from build123d import *

# Parameters (mm, degrees)
SKETCH_1_W                 = 300
SKETCH_1_H                 = 30
EXTRUDE_1_DEPTH            = 20
SKETCH_3_R                 = 4
CUT_EXTRUDE_1_DEPTH        = 155.272486205
SKETCH_3_3_R               = 6
SKETCH_3_3_R_2             = 4
CUT_EXTRUDE_2_DEPTH        = 155.272486205
SKETCH_3_4_R               = 13.5
SKETCH_3_4_R_2             = 13.25
SKETCH_3_4_R_3             = 6
CUT_EXTRUDE_3_DEPTH        = 155.272486205
SKETCH_3_5_R               = 2.4
CUT_EXTRUDE_4_DEPTH        = 4.5
SKETCH_3_6_R               = 2.4
CUT_EXTRUDE_5_DEPTH        = 5
SKETCH_4_R                 = 5
EXTRUDE_2_DEPTH            = 28
SKETCH_5_R                 = 2.55
CUT_EXTRUDE_6_DEPTH        = 4
SKETCH_6_W                 = 8.216991224
SKETCH_6_H                 = 30
CUT_EXTRUDE_7_DEPTH        = 5
CHAMFER_1_SIZE             = 2
CHAMFER_1_OF_MIRROR_2_SIZE = 2


with BuildPart() as part:
    # Sketch 1 → Extrude 1 (new body)
    with BuildSketch(Plane.XY):
        with Locations((0, 15)):
            Rectangle(SKETCH_1_W, SKETCH_1_H)
    extrude(amount=EXTRUDE_1_DEPTH)

    # Sketch 3 → Cut-Extrude 1 (cut, through all)
    with BuildSketch(Plane(origin=(0, 0, 0), x_dir=(-1, 0, 0), z_dir=(0, 0, -1))):
        with Locations((0, 15)):
            Circle(SKETCH_3_R)
    extrude(amount=-CUT_EXTRUDE_1_DEPTH, mode=Mode.SUBTRACT)

    # Sketch 3_3 → Cut-Extrude 2 (cut, through all)
    with BuildSketch(Plane(origin=(0, 0, 0), x_dir=(-1, 0, 0), z_dir=(0, 0, -1))):
        with Locations((0, 15)):
            Circle(SKETCH_3_3_R)
        with Locations((0, 15)):
            Circle(SKETCH_3_3_R_2, mode=Mode.SUBTRACT)
    extrude(amount=-CUT_EXTRUDE_2_DEPTH, mode=Mode.SUBTRACT)

    # Sketch 3_4 → Cut-Extrude 3 (cut, through all)
    # profile 1 of 2: a face of its own
    with BuildSketch(Plane(origin=(0, 0, 0), x_dir=(-1, 0, 0), z_dir=(0, 0, -1))):
        with Locations((0, 15)):
            Circle(SKETCH_3_4_R)
        with Locations((0, 15)):
            Circle(SKETCH_3_4_R_2, mode=Mode.SUBTRACT)
    # profile 2 of 2: a face of its own
    with BuildSketch(Plane(origin=(0, 0, 0), x_dir=(-1, 0, 0), z_dir=(0, 0, -1))):
        with Locations((0, 15)):
            Circle(SKETCH_3_4_R_2)
        with Locations((0, 15)):
            Circle(SKETCH_3_4_R_3, mode=Mode.SUBTRACT)
    extrude(amount=-CUT_EXTRUDE_3_DEPTH, mode=Mode.SUBTRACT)

    # Sketch 3_5 → Cut-Extrude 4 (cut)
    # profile 1 of 2: a face of its own
    with BuildSketch(Plane(origin=(0, 0, 0), x_dir=(-1, 0, 0), z_dir=(0, 0, -1))):
        with BuildLine():
            ThreePointArc((-6.02027027, 2.916691435), (-13.5, 15), (-6.02027027, 27.083308565))
            Line((-6.02027027, 27.083308565), (-20.841216216, 19.699064442))
            ThreePointArc((-20.841216216, 19.699064442), (-23.75, 15), (-20.841216216, 10.300935558))
            Line((-20.841216216, 10.300935558), (-6.02027027, 2.916691435))
        make_face()
        with Locations((-18.5, 15)):
            Circle(SKETCH_3_5_R, mode=Mode.SUBTRACT)
    # profile 2 of 2: a face of its own
    with BuildSketch(Plane(origin=(0, 0, 0), x_dir=(-1, 0, 0), z_dir=(0, 0, -1))):
        with BuildLine():
            Line((20.841216216, 19.699064442), (6.02027027, 27.083308565))
            ThreePointArc((6.02027027, 27.083308565), (11.478755347, 22.105503197), (13.5, 15))
            ThreePointArc((13.5, 15), (11.478755347, 7.894496803), (6.02027027, 2.916691435))
            Line((6.02027027, 2.916691435), (20.841216216, 10.300935558))
            ThreePointArc((20.841216216, 10.300935558), (23.75, 15), (20.841216216, 19.699064442))
        make_face()
        with Locations((18.5, 15)):
            Circle(SKETCH_3_5_R, mode=Mode.SUBTRACT)
    cut_extrude_4 = extrude(amount=-CUT_EXTRUDE_4_DEPTH, mode=Mode.SUBTRACT)

    # Sketch 3_6 → Cut-Extrude 5 (cut)
    with BuildSketch(Plane(origin=(0, 0, 0), x_dir=(-1, 0, 0), z_dir=(0, 0, -1))):
        with Locations((-18.5, 15)):
            Circle(SKETCH_3_6_R)
        with Locations((18.5, 15)):
            Circle(SKETCH_3_6_R)
    cut_extrude_5 = extrude(amount=-CUT_EXTRUDE_5_DEPTH, mode=Mode.SUBTRACT)

    # Sketch 4 → Extrude 2 (add)
    with BuildSketch(Plane.ZY.offset(150)):
        with Locations((10, 15)):
            Circle(SKETCH_4_R)
    extrude_2 = extrude(amount=EXTRUDE_2_DEPTH)

    # Mirror 1: Extrude 2 across plane
    add(extrude_2.mirror(Plane.ZY))

    # Sketch 5 → Cut-Extrude 6 (cut)
    with BuildSketch(Plane.XY.offset(20)):
        with Locations((-138, 15)):
            Circle(SKETCH_5_R)
    cut_extrude_6 = extrude(amount=-CUT_EXTRUDE_6_DEPTH, mode=Mode.SUBTRACT)

    # Sketch 6 → Cut-Extrude 7 (cut)
    with BuildSketch(Plane.XY.offset(16)):
        with Locations((-138, 15)):
            Rectangle(SKETCH_6_W, SKETCH_6_H)
    cut_extrude_7 = extrude(amount=-CUT_EXTRUDE_7_DEPTH, mode=Mode.SUBTRACT)

    # Chamfer 1
    chamfer_1_edges = [part.edges().sort_by_distance(p)[0] for p in [
        (-142.108495612, 30, 13.5),
        (-133.891504388, 30, 13.5),
        (-133.891504388, 0, 13.5),
        (-142.108495612, 0, 13.5),
    ]]
    chamfer(chamfer_1_edges, length=CHAMFER_1_SIZE)

    # Mirror 2: Cut-Extrude 6, Cut-Extrude 7 across plane
    add(cut_extrude_6.mirror(Plane.ZY), mode=Mode.SUBTRACT)
    add(cut_extrude_7.mirror(Plane.ZY), mode=Mode.SUBTRACT)

    # Chamfer 1 of Mirror 2
    chamfer_1_of_mirror_2_edges = [part.edges().sort_by_distance(p)[0] for p in [
        (142.108495612, 30, 13.5),
        (133.891504388, 30, 13.5),
        (133.891504388, 0, 13.5),
        (142.108495612, 0, 13.5),
    ]]
    chamfer(chamfer_1_of_mirror_2_edges, length=CHAMFER_1_OF_MIRROR_2_SIZE)

    # Mirror 3: Cut-Extrude 4, Cut-Extrude 5 across plane
    add(cut_extrude_4.mirror(Plane.XY.offset(10)), mode=Mode.SUBTRACT)
    add(cut_extrude_5.mirror(Plane.XY.offset(10)), mode=Mode.SUBTRACT)


solid = part.part
Could you check a few things on this model? Use its own coordinates, in mm. A direction names the side the tool comes from. Round coordinates to 2 decimals unless told otherwise and drop trailing zeros. Put each result on its own line as item: value. Start each with the question number.
(1) Will these pins go through, and if not, where does the flat tip stop? pin 1 (8 mm diameter, centred on y = 15.5, z = 4, fed in from -X); pin 2 (4.5 mm diameter, centred on x = 18.5, y = 15, fed in from -Z); pin 3 (6 mm diameter, centred on y = 5, z = 11.5, fed in from -X); pin 4 (5.5 mm diameter, centred on x = 18.5, y = 15, fed in from -Z).
(2) For faces 1 (the flat face through (-13.53, 23.34, 17.78)), 2 (the flat face through (-2, 0, 10)), 3 (the flat face through (15.6, 15.1, 4.5)), which set-ups out of +Z, -Z, +X, -X, +Y, -Y let a thin tool reach every point of the face, with its end or its side?
(3) Thinking about a two-plate mould opening in Y: for faces 4 (the flat face through (15.6, 15.1, 15.5)), 5 (the flat face through (-178, 15, 10)), 6 (the flat face through (-2, 30, 10)), 7 (the cylindrical face through (163.804, 10.564, 12.307)), which applies, released by +Y, released by -Y, zero draft, split by the parting line, or undercut?
(4) I need wall thicknesses on probe 1 along Y at (x, z) = (0, 12); probe 2 along Y at (x, z) = (-18.5, 4.8); probe 3 along X at (y, z) = (20, 12.5). Which ranges of each line are inside material? Lowest first, please.
Here are the results:
1. pin 1: stops at x = -178
1. pin 2: stops at z = 5
1. pin 3: stops at x = -150
1. pin 4: stops at z = 4.5
2. face 1: +Z
2. face 2: +Z, -Z, +X, -X, -Y
2. face 3: -Z
3. face 4: undercut
3. face 5: zero draft
3. face 6: released by +Y
3. face 7: split by the parting line
4. probe 1: y = 0 to 1.5, 28.5 to 30
4. probe 2: y = 0 to 12.6, 17.4 to 30
4. probe 3: x = -150 to -142.11, -133.89 to -12.54, 12.54 to 133.89, 142.11 to 150
